Can you work these out from the drawing? Everything is in mm from the part's minimum corner. A direction names the side the tool comes from. Coordinates: 2 decimals unless noted, no trailing zeros. Loops run counter-clockwise (first coordinate to the right, second up) from the corner with the lowest first, then second, coordinate; pieces in that order, holes last. Notation, with made-up numbers: (-24, 19) - (6, 19) arc R24 ccw to (6, 36) - close; hole circle Ø5 at (-27, 6.5). An arc over 180 degrees is marked (long way). Use CSV: the item, a comma, the result in double quotes.
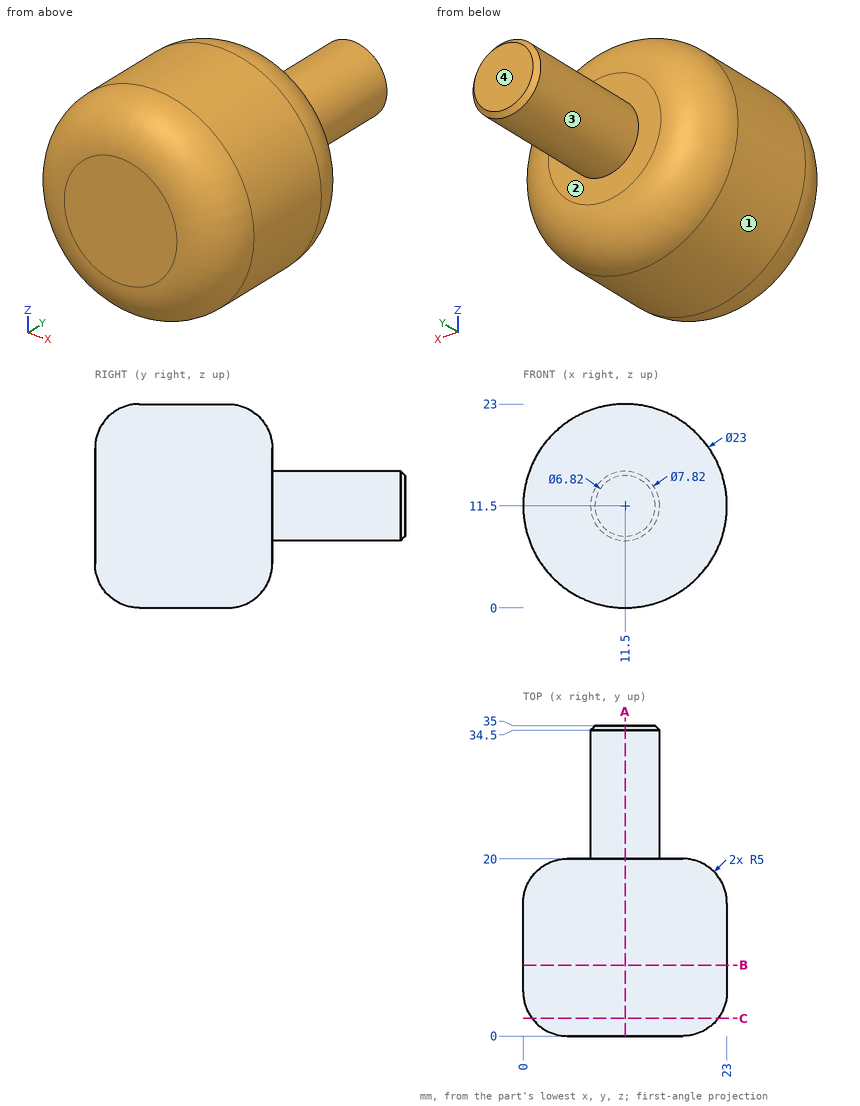
(1) Which directions (+Z, -Z, +X, -X, +Y, -Y) give clear straight access to the entire face, cutting with the end or side of a thin tool? Please do the marked faces 1 and 2.
Computed:
face 1,"+Y, -Y"
face 2,"+Y"
(2) Please list where these lines run through material, in increasing order: line 1 (Y direction, x = 7, z = 7.5); line 2 (Z direction, x = 11.5, y = 15); line 3 (X direction, y = 32, z = 11.25).
Computed:
line 1,"y = 0 to 20"
line 2,"z = 0 to 23"
line 3,"x = 7.6 to 15.4"
(3) Thinking about a two-plate mould opening in Z: for the marked faces 3 and 4, which applies, +Z half, -Z half, draft (parallel to the pull), parting line (faces both ways), or undercut?
Computed:
face 3,"parting line"
face 4,"draft"
(4) Suppose I cut it at B-B (y = 8). Write out the boundary of the cut face in (x, z).
Computed:
outline,"circle Ø23 at (11.5, 11.5)"
(5) Suppose I cut it at A-A (x = 11.5). Write out the boundary of the cut face in (y, z).
Computed:
outline,"(0, 5) arc R5 ccw to (5, 0) - (15, 0) arc R5 ccw to (20, 5) - (20, 7.59) - (34.5, 7.59) - (35, 8.09) - (35, 14.91) - (34.5, 15.41) - (20, 15.41) - (20, 18) arc R5 ccw to (15, 23) - (5, 23) arc R5 ccw to (0, 18) - close"
(6) Will these pins go through, and if not, where does the flat tip stop? pin 1 (8 mm diameter, centred on y = 6, z = 20.5, fed in from -X); pin 2 (8 mm diameter, centred on x = 19.5, y = 24.5, fed in from -Z); pin 3 (12 mm diameter, centred on x = 3, z = 14, fed in from -Y); pin 4 (10 mm diameter, centred on x = 5.5, y = 27.5, fed in from +Z).
Computed:
pin 1,"stops at x = 1.14"
pin 2,"passes through"
pin 3,"stops at y = 0"
pin 4,"stops at z = 15.28"
(7) Suppose I cut it at C-C (y = 2). Write out the boundary of the cut face in (x, z), plus the area to 3 significant figures.
Computed:
outline,"circle Ø21 at (11.5, 11.5)"
area,"346 mm²"
